```python
from build123d import *

# Parameters (mm, degrees)
BOSS_EXTRUDE2_DEPTH    = 30
SKETCH2_W              = 10
SKETCH2_H              = 190
CUT_EXTRUDE8_DEPTH     = 5
SKETCH7_W              = 10
SKETCH7_H              = 190
CUT_EXTRUDE9_DEPTH     = 5
SKETCH10_W             = 90
SKETCH10_H             = 20
BOSS_EXTRUDE9_DEPTH    = 30
SKETCH16_W             = 10
SKETCH16_H             = 5
CUT_EXTRUDE11_DEPTH    = 34
SKETCH18_W             = 10
SKETCH18_H             = 5
CUT_EXTRUDE12_DEPTH    = 36
SPLIT3_SURFACE_1_BACK  = 223.935
SPLIT3_SURFACE_1_DEPTH = 447.87
SPLIT3_SURFACE_2_BACK  = 223.935
SPLIT3_SURFACE_2_DEPTH = 447.87
SKETCH24_W             = 20
SKETCH24_H             = 30
BOSS_EXTRUDE10_DEPTH   = 5
SKETCH25_W             = 20
SKETCH25_H             = 30
BOSS_EXTRUDE11_DEPTH   = 5


with BuildPart() as part:
    # Sketch1 → Boss-Extrude2 (new body)
    with BuildSketch(Plane(origin=(0, 0, 0), x_dir=(1, 0, 0), z_dir=(0, 1, 0))):
        Polygon((10, 0), (10, 40), (0, 40), (0, 90), (10, 90), (10, 140), (0, 140), (0, 190), (100, 190), (100, 0), align=None)
    extrude(amount=BOSS_EXTRUDE2_DEPTH)

    # Sketch2 → Cut-Extrude8 (cut)
    with BuildSketch(Plane(origin=(0, 30, 0), x_dir=(1, 0, 0), z_dir=(0, 1, 0))):
        with Locations((27, 95)):
            Rectangle(SKETCH2_W, SKETCH2_H)
    extrude(amount=-CUT_EXTRUDE8_DEPTH, mode=Mode.SUBTRACT)

    # Sketch7 → Cut-Extrude9 (cut)
    with BuildSketch(Plane(origin=(0, 30, 0), x_dir=(1, 0, 0), z_dir=(0, 1, 0))):
        with Locations((83, 95)):
            Rectangle(SKETCH7_W, SKETCH7_H)
    extrude(amount=-CUT_EXTRUDE9_DEPTH, mode=Mode.SUBTRACT)

    # Sketch10 → Boss-Extrude9 (add)
    with BuildSketch(Plane(origin=(0, 30, 0), x_dir=(1, 0, 0), z_dir=(0, 1, 0))):
        with Locations((55, 110)):
            Rectangle(SKETCH10_W, SKETCH10_H)
    extrude(amount=BOSS_EXTRUDE9_DEPTH)

    # Sketch16 → Cut-Extrude11 (cut)
    with BuildSketch(Plane(origin=(0, 0, -120), x_dir=(-1, 0, 0), z_dir=(0, 0, -1))):
        with Locations((-83, 32.5)):
            Rectangle(SKETCH16_W, SKETCH16_H)
    extrude(amount=-CUT_EXTRUDE11_DEPTH, mode=Mode.SUBTRACT)

    # Sketch18 → Cut-Extrude12 (cut)
    with BuildSketch(Plane(origin=(0, 0, -120), x_dir=(-1, 0, 0), z_dir=(0, 0, -1))):
        with Locations((-27, 32.5)):
            Rectangle(SKETCH18_W, SKETCH18_H)
    extrude(amount=-CUT_EXTRUDE12_DEPTH, mode=Mode.SUBTRACT)


with BuildPart() as body_2:
    # Split3: the piece behind the surface
    add(part.part)
    # Split3 surface: a surface, the sketch's curves swept straight by 447.87 mm
    with BuildLine(Plane.ZY.offset(-10).offset(-SPLIT3_SURFACE_1_BACK), mode=Mode.PRIVATE) as split3_surface_1_path:
        Line((-120, 30), (-100, 30))
    split3_surface_1 = Shell.extrude(split3_surface_1_path.wire(), (-1 * SPLIT3_SURFACE_1_DEPTH, 0 * SPLIT3_SURFACE_1_DEPTH, 0 * SPLIT3_SURFACE_1_DEPTH))
    split(bisect_by=split3_surface_1, keep=Keep.BOTTOM)


with BuildPart() as part_1:
    add(part.part)

    # Split3: split by a surface, the side it looks to stays
    # Split3 surface: a surface, the sketch's curves swept straight by 447.87 mm
    with BuildLine(Plane.ZY.offset(-10).offset(-SPLIT3_SURFACE_2_BACK), mode=Mode.PRIVATE) as split3_surface_2_path:
        Line((-120, 30), (-100, 30))
    split3_surface_2 = Shell.extrude(split3_surface_2_path.wire(), (-1 * SPLIT3_SURFACE_2_DEPTH, 0 * SPLIT3_SURFACE_2_DEPTH, 0 * SPLIT3_SURFACE_2_DEPTH))
    split(bisect_by=split3_surface_2, keep=Keep.TOP)

    add(body_2.part)  # Boss-Extrude10 merges body 2
    # Sketch24 → Boss-Extrude10 (add)
    with BuildSketch(Plane.ZY.offset(-10)):
        with Locations((-110, 45)):
            Rectangle(SKETCH24_W, SKETCH24_H)
    extrude(amount=BOSS_EXTRUDE10_DEPTH)

    # Sketch25 → Boss-Extrude11 (add)
    with BuildSketch(Plane(origin=(100, 0, 0), x_dir=(0, 0, -1), z_dir=(1, 0, 0))):
        with Locations((110, 45)):
            Rectangle(SKETCH25_W, SKETCH25_H)
    extrude(amount=BOSS_EXTRUDE11_DEPTH)


solid = part_1.part
```
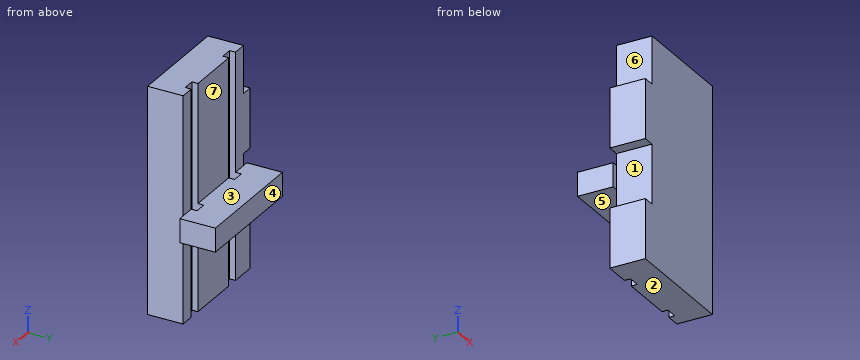
The listing builds one solid part. Answer for the finished solid, in the listing's coordinates (mm). Face numbers are marked on the shaded views. A direction names the side the tool comes from. Coordinates: 2 decimals unless noted, no trailing zeros. Write each loop counter-clockwise with the first axis right and the second up, starting at its lowest first coordinate (ties: lowest second). Pieces come first, ordered by that corner, then holes. Notation, with made-up numbers: M 87,77.5 L 95,77.5 A10 cw 95,91.5 Z; hole C -32,48 d8. An arc over 180 degrees is marked long. Use a Markdown table: item, result. Add a question column.
1. Straight lines are drawn through the part: line 1 along X through (y, z) = (28.5, -41); line 2 along X through (y, z) = (5.5, -98); line 3 along Y through (x, z) = (66, -80.5). For each, find the intervals that lie inside material, in ascending order. Write a range as [from, to].
2. Section A-A (x = 80) is taken. Give the vertices of the cut face in (y, z), plus the area to 3 significant figures.
3. Section D-D (x = 50.5) is taken. Give the vertices of the cut face in (y, z).
4. Section B-B (z = -116.5) is taken. Give the vertices of the cut face in (x, y), plus the area to 3 significant figures.
5. For a pull along Z with two mould halves and no side action, classify the marked faces 1, 2 and 3 as +Z half, -Z half, draft (parallel to the pull), parting line (faces both ways), or undercut.
6. Section C-C (y = 17) is taken. Give the vertices of the cut face in (x, z).
7. Given P1, Ø10, axis at x = 75.5, y = 47, coming from the +Z side; P2, Ø3, axis at x = 27.5, z = -140.5, coming from the +Y side; P3, Ø1, axis at y = 26, z = -145, coming from the +X side; P4, Ø1.5, axis at y = 31, z = -26, coming from the +X side, each flat-ended and moving along its own axis, determine where each tip first touches the part or whether it passes through.
8. Which of the six approach directions +Z, -Z, +X, -X, +Y, -Y give full straight-line access (tool end or side, diameter ignored) to the marked faces 4, 5, 6 and 7?
Data:
| question | item | result |
|---|---|---|
| 1 | line 1 | x = [0, 22], [32, 78], [88, 100] |
| 1 | line 2 | x = [10, 100] |
| 1 | line 3 | y = [0, 30] |
| 2 | outline | M 0,-190 L 25,-190 L 25,0 L 0,0 Z; M 35,-120 L 60,-120 L 60,-100 L 35,-100 Z |
| 2 | area | 5,250 mm2 |
| 3 | outline | M 0,-190 L 30,-190 L 30,-120 L 60,-120 L 60,-100 L 30,-100 L 30,0 L 0,0 Z |
| 4 | outline | M 5,30 L 10,30 L 10,0 L 100,0 L 100,30 L 105,30 L 105,60 L 5,60 Z; hole M 22,25 L 32,25 L 32,35 L 22,35 Z; hole M 78,25 L 88,25 L 88,35 L 78,35 Z |
| 4 | area | 5,500 mm2 |
| 5 | face 1 | undercut |
| 5 | face 2 | -Z half |
| 5 | face 3 | +Z half |
| 6 | outline | M 0,-190 L 100,-190 L 100,0 L 10,0 L 10,-40 L 0,-40 L 0,-90 L 10,-90 L 10,-140 L 0,-140 Z |
| 7 | P1 | stops at z = -100 |
| 7 | P2 | stops at y = 25 |
| 7 | P3 | stops at x = 100 |
| 7 | P4 | passes through |
| 8 | face 4 | +Z, -Z, +X, -X, +Y |
| 8 | face 5 | -Z, +X, -X, +Y |
| 8 | face 6 | +Z, -X, +Y, -Y |
| 8 | face 7 | +Z, +X, -X, +Y |
